Read the model definition and answer for the solid it produces. Units are mm, in the model's axes. A direction names the side the tool comes from. Coordinates: 2 decimals unless noted, no trailing zeros. Order: outer loops, then holes, each group sorted by start corner. A loop starts at its lowest first (then second) coordinate and runs counter-clockwise, first axis right, second up. Notation, with made-up numbers: (55, 88.5) -> (99, 88.5) arc R31 cw to (99, 124.5) -> close; hole circle Ø8 at (55.25, -26.5). An arc over 180 degrees is marked (long way). Answer in a Markdown table with one row per item.
from build123d import *

# Parameters (mm, degrees)
SKETCH_1_R      = 6.7
EXTRUDE_1_DEPTH = 10
SKETCH_1_5_R    = 2.925
EXTRUDE_2_DEPTH = 6
CHAMFER_1_SIZE  = 1
FILLET_1_R      = 0.4
FILLET_2_R      = 2


with BuildPart() as part:
    # Sketch 1 → Extrude 1 (new body)
    with BuildSketch(Plane(origin=(0, 0, 0), x_dir=(1, 0, 0), z_dir=(0, 1, 0))):
        with Locations(Location((0, 0, 0), (0, 0, 270))):
            Circle(SKETCH_1_R)
    extrude(amount=EXTRUDE_1_DEPTH)

    # Sketch 1_5 → Extrude 2 (add)
    with BuildSketch(Plane(origin=(0, 0, 0), x_dir=(1, 0, 0), z_dir=(0, 1, 0))):
        with Locations(Location((0, 0, 0), (0, 0, 270))):
            Circle(SKETCH_1_5_R)
    extrude(amount=-EXTRUDE_2_DEPTH)

    # Chamfer 1
    chamfer_1_edges = [part.edges().sort_by_distance(p)[0] for p in [
        (0, 0, -6.7),
        (0, -6, -2.925),
    ]]
    chamfer(chamfer_1_edges, length=CHAMFER_1_SIZE)

    # Fillet 1
    fillet_1_edges = [part.edges().sort_by_distance(p)[0] for p in [
        (0, 0, -2.925),
    ]]
    fillet(fillet_1_edges, radius=FILLET_1_R)

    # Fillet 2
    fillet_2_edges = [part.edges().sort_by_distance(p)[0] for p in [
        (0, 10, -6.7),
    ]]
    fillet(fillet_2_edges, radius=FILLET_2_R)


solid = part.part
Q1. The part is cut by section B-B (x = 0). Write down the section's boundary in (y, z) (3 decimals), then the cut area to 3 significant figures.
Outcome:
| item | result |
|---|---|
| outline | (-6, -1.925) -> (-5, -2.925) -> (-0.4, -2.925) arc R0.4 cw to (0, -3.325) -> (0, -5.7) -> (1, -6.7) -> (8, -6.7) arc R2 ccw to (10, -4.7) -> (10, 4.7) arc R2 ccw to (8, 6.7) -> (1, 6.7) -> (0, 5.7) -> (0, 3.325) arc R0.4 cw to (-0.4, 2.925) -> (-5, 2.925) -> (-6, 1.925) -> close |
| area | 165 mm² |
Q2. The part is cut by section A-A (z = 0). Write down the section's boundary in (x, y) (3 decimals).
Outcome:
| item | result |
|---|---|
| outline | (-6.7, 1) -> (-5.7, 0) -> (-3.325, 0) arc R0.4 cw to (-2.925, -0.4) -> (-2.925, -5) -> (-1.925, -6) -> (1.925, -6) -> (2.925, -5) -> (2.925, -0.4) arc R0.4 cw to (3.325, 0) -> (5.7, 0) -> (6.7, 1) -> (6.7, 8) arc R2 ccw to (4.7, 10) -> (-4.7, 10) arc R2 ccw to (-6.7, 8) -> close |
Q3. Consider line 1 (Y direction, x = -2.5, z = 3.75); line 2 (X direction, y = -0.25, z = -2.25); line 3 (X direction, y = 4, z = -2.75). Determine where each line is inside the solid, lowest interval first.
Outcome:
| item | result |
|---|---|
| line 1 | 0 to 10 |
| line 2 | -1.91 to 1.91 |
| line 3 | -6.11 to 6.11 |
Q4. The part is cut by section C-C (y = -2.5). Write down the section's boundary in (x, z) (3 decimals), then the cut area to 3 significant figures.
Outcome:
| item | result |
|---|---|
| outline | circle Ø5.85 at (0, 0) |
| area | 26.9 mm² |
Q5. Given pin 1 (3 mm diameter, centred on x = -5.5, y = -0.5, fed in from +Z); pin 2 (1.5 mm diameter, centred on x = -1, y = 7, fed in from -Z), each flat-ended and moving along its own axis, determine where each tip first touches the part or whether it passes through.
Outcome:
| item | result |
|---|---|
| pin 1 | z = 4.45 |
| pin 2 | z = -6.7 |
Q6. For faces 1 (the face through (0, -6, 0)), 2 (the face through (-2.5, 0, 2.5)), determine the directions among +Z, -Z, +X, -X, +Y, -Y from which every point of the face is accessible in a straight line to the end or side of a thin tool.
Outcome:
| item | result |
|---|---|
| face 1 | +Z, -Z, +X, -X, -Y |
| face 2 | -Y |
Q7. The part is cut by section D-D (y = 1.75). Write down the section's boundary in (x, z).
Outcome:
| item | result |
|---|---|
| outline | circle Ø13.4 at (0, 0) |
